Could you check a few things on this model? Use its own coordinates, in mm. Face numbers are marked on the shaded views. Coordinates: 2 decimals unless noted, no trailing zeros. Loops run counter-clockwise (first coordinate to the right, second up) from the corner with the lowest first, then second, coordinate; pieces in that order, holes last.
1) Imagine slicing it at B-B on y = 3. Please give me the cut outline in (x, z).
2) Imagine slicing it at C-C on z = 0.35. Please give me the cut outline in (x, y) (3 decimals), plus the area to 3 significant figures.
3) Imagine slicing it at D-D on x = 3.25. Please give me the cut outline in (y, z) (3 decimals).
4) If I drill on line 1 along X through (y, z) = (0.5, 0.1); line 2 along X through (y, z) = (3.25, 0.2); line 3 along Y through (x, z) = (4, 0.75), over which ranges is the centre line in solid material (lowest first)?
5) Will this pin go through, and if not, where does the flat tip stop? P1, Ø5, axis at x = 2.5, y = -3, coming from the -Z side.
6) Imagine slicing it at A-A on x = 0. Please give me the cut outline in (y, z).
7) Thinking about a two-plate mould opening in X: for the marked faces 1, 2 and 3, which applies, released by +X, released by -X, zero draft, split by the parting line, or undercut?
```python
from build123d import *

# Parameters (mm, degrees)
SKETCH_1_W          = 12
SKETCH_1_H          = 10
EXTRUDE_1_DEPTH     = 0.8
CUT_EXTRUDE_1_REACH = 9.851
SKETCH_2_R          = 2
SKETCH_2_R_2        = 0.75
SKETCH_2_R_3        = 0.375
FILLET_1_R          = 1


with BuildPart() as part:
    # Эскиз1 → Бобышка-Вытянуть1 (new body)
    with BuildSketch(Plane.XY):
        Rectangle(SKETCH_1_W, SKETCH_1_H)
    extrude(amount=EXTRUDE_1_DEPTH)

    # Эскиз2 → Вырез-Вытянуть1 (cut, up to next)
    with BuildSketch(Plane.XY.offset(0.8), mode=Mode.PRIVATE) as cut_extrude_1_sk1:
        Circle(SKETCH_2_R)
    cut_extrude_1_tool1 = extrude(cut_extrude_1_sk1.sketch, amount=-CUT_EXTRUDE_1_REACH, mode=Mode.PRIVATE) & part.part
    # Эскиз2 → Вырез-Вытянуть1 (cut, up to next)
    with BuildSketch(Plane.XY.offset(0.8), mode=Mode.PRIVATE) as cut_extrude_1_sk2:
        with Locations((-3.6, -3)):
            Circle(SKETCH_2_R_2)
    cut_extrude_1_tool2 = extrude(cut_extrude_1_sk2.sketch, amount=-CUT_EXTRUDE_1_REACH, mode=Mode.PRIVATE) & part.part
    # Эскиз2 → Вырез-Вытянуть1 (cut, up to next)
    with BuildSketch(Plane.XY.offset(0.8), mode=Mode.PRIVATE) as cut_extrude_1_sk3:
        with Locations((3.6, 3)):
            Circle(SKETCH_2_R_2)
    cut_extrude_1_tool3 = extrude(cut_extrude_1_sk3.sketch, amount=-CUT_EXTRUDE_1_REACH, mode=Mode.PRIVATE) & part.part
    # Эскиз2 → Вырез-Вытянуть1 (cut, up to next)
    with BuildSketch(Plane.XY.offset(0.8), mode=Mode.PRIVATE) as cut_extrude_1_sk4:
        with Locations((3.25, -2)):
            Circle(SKETCH_2_R_3)
    cut_extrude_1_tool4 = extrude(cut_extrude_1_sk4.sketch, amount=-CUT_EXTRUDE_1_REACH, mode=Mode.PRIVATE) & part.part
    add(cut_extrude_1_tool1.solids().sort_by_distance((0, 0, 0.8))[0], mode=Mode.SUBTRACT)
    add(cut_extrude_1_tool2.solids().sort_by_distance((-3.6, -3, 0.8))[0], mode=Mode.SUBTRACT)
    add(cut_extrude_1_tool3.solids().sort_by_distance((3.6, 3, 0.8))[0], mode=Mode.SUBTRACT)
    add(cut_extrude_1_tool4.solids().sort_by_distance((3.25, -2, 0.8))[0], mode=Mode.SUBTRACT)

    # Скругление1
    fillet_1_edges = [part.edges().sort_by_distance(p)[0] for p in [
        (6, -5, 0.4),
        (-6, -5, 0.4),
        (-6, 5, 0.4),
        (6, 5, 0.4),
    ]]
    fillet(fillet_1_edges, radius=FILLET_1_R)


solid = part.part
```
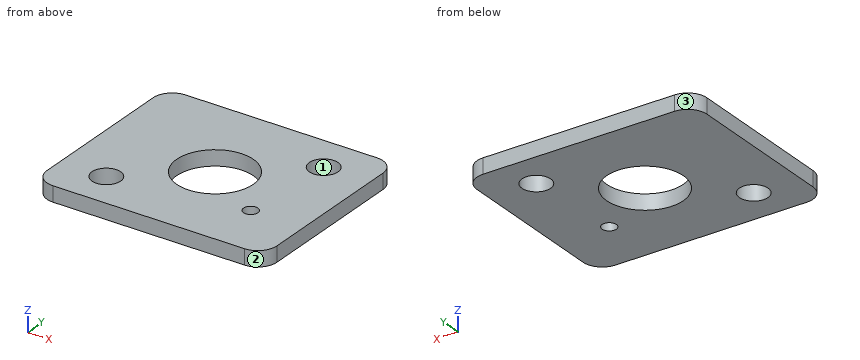
Filled in:
1. outline: (-6, 0) - (2.85, 0) - (2.85, 0.8) - (-6, 0.8) - close; (4.35, 0) - (6, 0) - (6, 0.8) - (4.35, 0.8) - close
2. outline: (-6, -4) arc R1 ccw to (-5, -5) - (5, -5) arc R1 ccw to (6, -4) - (6, 4) arc R1 ccw to (5, 5) - (-5, 5) arc R1 ccw to (-6, 4) - close; hole circle Ø1.5 at (-3.6, -3); hole circle Ø4 at (0, 0); hole circle Ø1.5 at (3.6, 3); hole circle Ø0.75 at (3.25, -2)
2. area: 103 mm2
3. outline: (-5, 0) - (-2.375, 0) - (-2.375, 0.8) - (-5, 0.8) - close; (-1.625, 0) - (2.337, 0) - (2.337, 0.8) - (-1.625, 0.8) - close; (3.663, 0) - (5, 0) - (5, 0.8) - (3.663, 0.8) - close
4. line 1: x = -6 to -1.94, 1.94 to 6
4. line 2: x = -6 to 2.89, 4.31 to 6
4. line 3: y = -5 to 2.37, 3.63 to 5
5. P1: stops at z = 0
6. outline: (-5, 0) - (-2, 0) - (-2, 0.8) - (-5, 0.8) - close; (2, 0) - (5, 0) - (5, 0.8) - (2, 0.8) - close
7. face 1: undercut
7. face 2: released by +X
7. face 3: released by -X
